from build123d import *

# Parameters (mm, degrees)
CUT_EXTRUDE_1_DEPTH = 1.1
FILLET_1_R          = 0.2


with BuildPart() as part:
    # 草图1 → 旋转1 (revolve)
    with BuildSketch(Plane.XY):
        Polygon((0, 0), (0, 2.25), (2.43, 2.25), (2.43, 1.25), (47.43, 1.25), (47.43, 0), align=None)
    revolve(axis=Axis((0, 0, 0), (1, 0, 0)))

    # 草图2 → 切除-拉伸1 (cut)
    with BuildSketch(Plane.ZY):
        Polygon((-1.154700538, 0), (-0.577350269, -1), (0.577350269, -1), (1.154700538, 0), (0.577350269, 1), (-0.577350269, 1), align=None)
    extrude(amount=-CUT_EXTRUDE_1_DEPTH, mode=Mode.SUBTRACT)

    # 圆角1
    fillet_1_edges = [part.edges().sort_by_distance(p)[0] for p in [
        (0, -2.25, 0),
    ]]
    fillet(fillet_1_edges, radius=FILLET_1_R)


solid = part.part
Build history of the part. All positions in model axes, mm. A direction names the side the tool comes from. Coordinates: 2 decimals unless noted, no trailing zeros. Write each loop counter-clockwise with the first axis right and the second up, starting at its lowest first coordinate (ties: lowest second). Pieces come first, ordered by that corner, then holes.
(1) Mould opens along Z. For faces 1 (the cylindrical face through (1.33, -0.29, 2.23)), 2 (the flat face through (0.54, -0.49, -0.87)), 3 (the flat face through (2.43, 1, -1)) say: pulls with the +Z half, pulls with the -Z half, needs draft (parallel to the pull), parting line crosses it, or undercut.
(2) 3-axis set-ups, long thin cutter, end or side, ignore diameter. For faces 4 (the flat face through (1.1, 0, 0)), 5 (the flat face through (47.43, 0, 0)), 6 (the cylindrical face through (25.24, -0.27, -1.22)): which of +Z, -Z, +X, -X, +Y, -Y reach the whole face in a straight line?
(3) Drill centre lines: line 1 (X direction, y = -0.6, z = 0.45); line 2 (Z direction, x = 33, y = -0.75); line 3 (X direction, y = 1.1, z = 1.1). Where is each one in solid material? Low to high.
(4) Cut at B-B on x = 15.5. List the corners of the cut face in (y, z), and give its area (3 significant figures).
(5) Pin check, flat tips, straight feed: pin 1 Ø1.5 at (x, y) = (5, 1.5) entering from +Z; pin 2 Ø1.5 at (x, y) = (32.5, -0.5) entering from -Z; pin 3 Ø0.6 at (y, z) = (0, 0.5) entering from -X. Stop position of each tip, or through.
(6) Cut at A-A on z = 0. List the corners of the cut face in (x, y).
Working result:
1. face 1: parting line crosses it
1. face 2: undercut
1. face 3: needs draft
2. face 4: -X
2. face 5: +Z, -Z, +X, +Y, -Y
2. face 6: +X
3. line 1: x = 1.1 to 47.43
3. line 2: z = -1 to 1
3. line 3: x = 0 to 2.43
4. outline: circle Ø2.5 at (0, 0)
4. area: 4.91 mm2
5. pin 1: stops at z = 1
5. pin 2: stops at z = -1.25
5. pin 3: stops at x = 1.1
6. outline: (0, -2.05) arc R0.2 ccw to (0.2, -2.25) - (2.43, -2.25) - (2.43, -1.25) - (47.43, -1.25) - (47.43, 1.25) - (2.43, 1.25) - (2.43, 2.25) - (0.2, 2.25) arc R0.2 ccw to (0, 2.05) - (0, 1) - (1.1, 1) - (1.1, -1) - (0, -1) - close
